Verification items for the finished model (mm, model axes). Face numbers are marked on the shaded views. Round coordinates to 2 decimals unless told otherwise and drop trailing zeros. Order: outer loops, then holes, each group sorted by start corner. A loop starts at its lowest first (then second) coordinate and runs counter-clockwise, first axis right, second up.
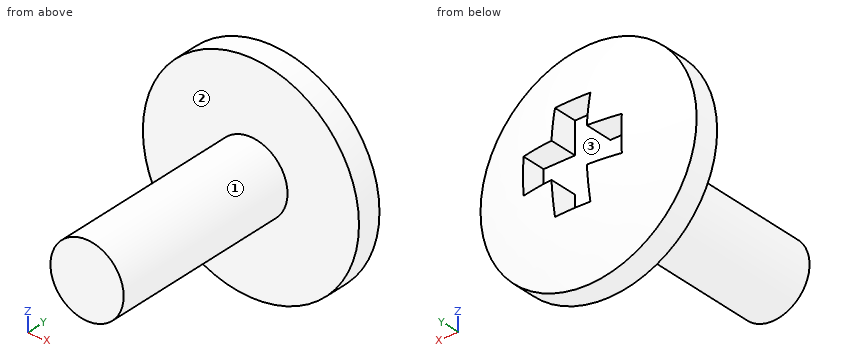
```python
from build123d import *

# Parameters (mm, degrees)
EXTRUDE1_DEPTH = 2.54


with BuildPart() as part:
    # Sketch1 → Revolve1 (revolve)
    with BuildSketch(Plane.XY):
        with BuildLine():
            Line((0, 0), (0, -6.35))
            Line((0, -6.35), (0.946564988, -6.35))
            Line((0.946564988, -6.35), (0.946564988, -1.27))
            Line((0.946564988, -1.27), (2.794, -1.27))
            Line((2.794, -1.27), (2.794, -0.635))
            ThreePointArc((2.794, -0.635), (1.4326253, -0.16074868), (0, 0))
        make_face()
    revolve(axis=Axis((0, 0, 0), (0, -1, 0)))

    # Sketch2 → Extrude1 (cut)
    with BuildSketch(Plane.XZ.offset(0.762)):
        Polygon((0.4572, -1.27), (-0.4572, -1.27), (-0.4572, -0.4572), (-1.27, -0.4572), (-1.27, 0.4572), (-0.4572, 0.4572), (-0.4572, 1.27), (0.4572, 1.27), (0.4572, 0.4572), (1.27, 0.4572), (1.27, -0.4572), (0.4572, -0.4572), align=None)
    extrude(amount=-EXTRUDE1_DEPTH, mode=Mode.SUBTRACT)


solid = part.part
```
1) Sectioned sample at C-C on y = -5.5. Record the cut outline in (x, z).
2) Scan lines: probe 1 along Z at (x, y) = (-0.05, -5); probe 2 along Y at (x, z) = (0.45, 0.4); probe 3 along Z at (x, y) = (-0.45, -4). Record each from-to range of solid material in increasing order.
3) Sectioned sample at D-D on z = 1.7. Record the cut outline in (x, y) (3 decimals).
4) Sectioned sample at B-B on x = 0. Record the cut outline in (y, z) (3 decimals), then the cut area to 3 significant figures.
5) Go/stop test with flat-tipped pins: pin 1 Ø2 at (y, z) = (-1.5, 0.5) entering from -X; pin 2 Ø0.8 at (y, z) = (-0.5, 1) entering from +X; pin 3 Ø0.6 at (y, z) = (-0.5, -1) entering from -X; pin 4 Ø0.6 at (x, y) = (-0.5, -0.5) entering from +Z. Record where each tip stops, or that it passes through.
6) Draft check along X on the marked faces 1, 2 and 3. Enter one of: released by +X, released by -X, zero draft, split by the parting line, or undercut.
7) Sectioned sample at A-A on z = 0. Record the cut outline in (x, y) (3 decimals).
Returned:
1. outline: circle Ø1.89 at (0, 0)
2. probe 1: z = -0.95 to 0.95
2. probe 2: y = -6.35 to -0.76
2. probe 3: z = -0.83 to 0.83
3. outline: (-2.217, -1.27) - (2.217, -1.27) - (2.217, -0.635) arc R6.237 ccw to (-2.217, -0.635) - close
4. outline: (-6.35, -0.947) - (-1.27, -0.947) - (-1.27, -2.794) - (-0.635, -2.794) arc R6.464 ccw to (-0.126, -1.27) - (-0.762, -1.27) - (-0.762, 1.27) - (-0.126, 1.27) arc R6.464 ccw to (-0.635, 2.794) - (-1.27, 2.794) - (-1.27, 0.947) - (-6.35, 0.947) - close
4. area: 13.7 mm2
5. pin 1: stops at x = -2.79
5. pin 2: stops at x = 2.72
5. pin 3: stops at x = -2.7
5. pin 4: stops at z = 2.78
6. face 1: split by the parting line
6. face 2: zero draft
6. face 3: undercut
7. outline: (-2.794, -1.27) - (-0.947, -1.27) - (-0.947, -6.35) - (0.947, -6.35) - (0.947, -1.27) - (2.794, -1.27) - (2.794, -0.635) arc R6.464 ccw to (1.27, -0.126) - (1.27, -0.762) - (-1.27, -0.762) - (-1.27, -0.126) arc R6.464 ccw to (-2.794, -0.635) - close
